The model under review builds one solid part; all positions refer to its coordinate system, in mm. Face numbers are marked on the shaded views. A direction names the side the tool comes from. Give positions to 0.01 mm unless a question says otherwise; leave off trailing zeros. Order: outer loops, then holes, each group sorted by start corner. A loop starts at its lowest first (then second) coordinate and runs counter-clockwise, first axis right, second up. Notation, with made-up numbers: (48.25, -24.75) - (71.25, -24.75) arc R38 cw to (71.25, 14.25) - close; hole circle Ø9 at (-14, 19). An arc over 180 degrees is marked (long way). Write item = value, one per line. Start each with the question number.
1. Mouldability with a two-part tool opening along X and no side actions: class the marked faces 4, 5, 6 and 7 as pulls with the +X half, pulls with the -X half, needs draft (parallel to the pull), parting line crosses it, or undercut.
2. We need section D-D, the plane x = 0. Give the boundary of the cut face in (y, z).
3. Wall thickness on probe 1 along Z at (x, y) = (-24, -14.8); probe 2 along X at (y, z) = (-14, 0.5); probe 3 along X at (y, z) = (-8.5, 8): over which ranges is each line inside the solid? List them lowest first.
4. Machinability: for the marked faces 1, 2 and 3, which of the approach directions +Z, -Z, +X, -X, +Y, -Y give a long, thin tool a straight path to every point of the face, cutting with its end or side? Answer none if there is none.
5. We need section B-B, the plane z = 5. Give the boundary of the cut face in (x, y).
6. For P1, Ø5, axis at x = 19, z = 3.5, coming from the +Y side; P2, Ø6, axis at x = 0, z = 2, coming from the -Y side; P3, Ø1.5, axis at y = 4, z = 3, coming from the +X side; P4, Ø2.5, axis at x = -24, z = 5, coming from the +Y side, all flat-tipped, find the tip position at first contact; note any pin that passes through.
7. We need section A-A, the plane x = -24. Give the boundary of the cut face in (y, z).
8. We need section C-C, the plane y = 2. Give the boundary of the cut face in (x, z), and give its area (3 significant figures).
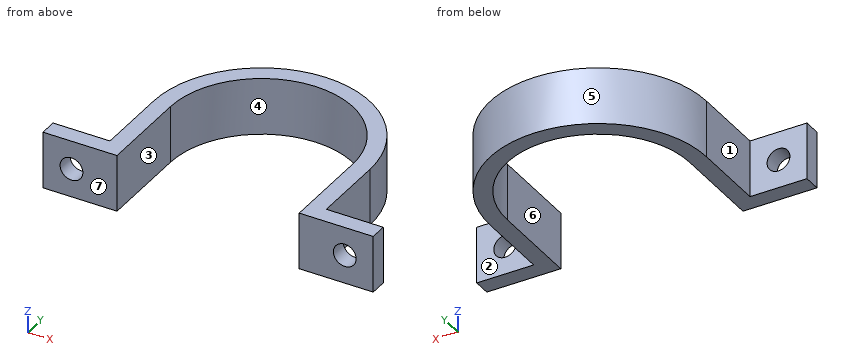
from build123d import *

# Parameters (mm, degrees)
CYLINDER001_R     = 2
CYLINDER001_DEPTH = 10
CYLINDER_R        = 2
CYLINDER_DEPTH    = 10
EXTRUDE_DEPTH     = 10


with BuildPart() as cylinder001:
    # Cylinder001 → Cylinder001 (new body)
    with BuildSketch(Plane(origin=(-24, -19, 5), x_dir=(1, 0, 0), z_dir=(0, 1, 0))):
        Circle(CYLINDER001_R)
    extrude(amount=CYLINDER001_DEPTH)


with BuildPart() as cylinder:
    # Cylinder → Cylinder (new body)
    with BuildSketch(Plane(origin=(24, -19, 5), x_dir=(1, 0, 0), z_dir=(0, 1, 0))):
        Circle(CYLINDER_R)
    extrude(amount=CYLINDER_DEPTH)


with BuildPart() as cut001:
    # Sketch → Extrude (new body)
    with BuildSketch(Plane.XY):
        with BuildLine():
            ThreePointArc((19, 0), (0, 19), (-19, 0))
            Line((-19, 0), (-19, -13))
            Line((-19, -13), (-29, -13))
            Line((-29, -13), (-29, -16))
            Line((-29, -16), (-16, -16))
            Line((-16, -16), (-16, 0))
            ThreePointArc((16, 0), (0, 16), (-16, 0))
            Line((16, -16), (16, 0))
            Line((29, -16), (16, -16))
            Line((29, -13), (29, -16))
            Line((19, -13), (29, -13))
            Line((19, 0), (19, -13))
        make_face()
    extrude(amount=EXTRUDE_DEPTH)

    # Cut: cut Cylinder
    add(cylinder.part, mode=Mode.SUBTRACT)

    # Cut001: cut Cylinder001
    add(cylinder001.part, mode=Mode.SUBTRACT)


solid = cut001.part
Model answer:
q1.face_4 = undercut
q1.face_5 = parting line crosses it
q1.face_6 = undercut
q1.face_7 = needs draft
q2.outline = (16, 0) - (19, 0) - (19, 10) - (16, 10) - close
q3.probe_1 = 0 to 3, 7 to 10
q3.probe_2 = -29 to -16, 16 to 29
q3.probe_3 = -19 to -16, 16 to 19
q4.face_1 = +Z, -Z, -X, +Y
q4.face_2 = +Z, -Z, +X, +Y
q4.face_3 = +Z, -Z, -Y
q5.outline = (-29, -16) - (-26, -16) - (-26, -13) - (-29, -13) - close; (-22, -16) - (-16, -16) - (-16, 0) arc R16 cw to (16, 0) - (16, -16) - (22, -16) - (22, -13) - (19, -13) - (19, 0) arc R19 ccw to (-19, 0) - (-19, -13) - (-22, -13) - close; (26, -16) - (29, -16) - (29, -13) - (26, -13) - close
q6.P1 = 9.42
q6.P2 = 15.72
q6.P3 = 18.72
q6.P4 = through
q7.outline = (-16, 0) - (-13, 0) - (-13, 3) - (-16, 3) - close; (-16, 7) - (-13, 7) - (-13, 10) - (-16, 10) - close
q8.outline = (-18.89, 0) - (-15.87, 0) - (-15.87, 10) - (-18.89, 10) - close; (15.87, 0) - (18.89, 0) - (18.89, 10) - (15.87, 10) - close
q8.area = 60.4 mm2
